Part print with two shaded views. Sizes in mm from the minimum x, y, z corner. Coordinates: 2 decimals unless noted, no trailing zeros. Order: outer loops, then holes, each group sorted by start corner. A loop starts at its lowest first (then second) coordinate and runs counter-clockwise, first axis right, second up.
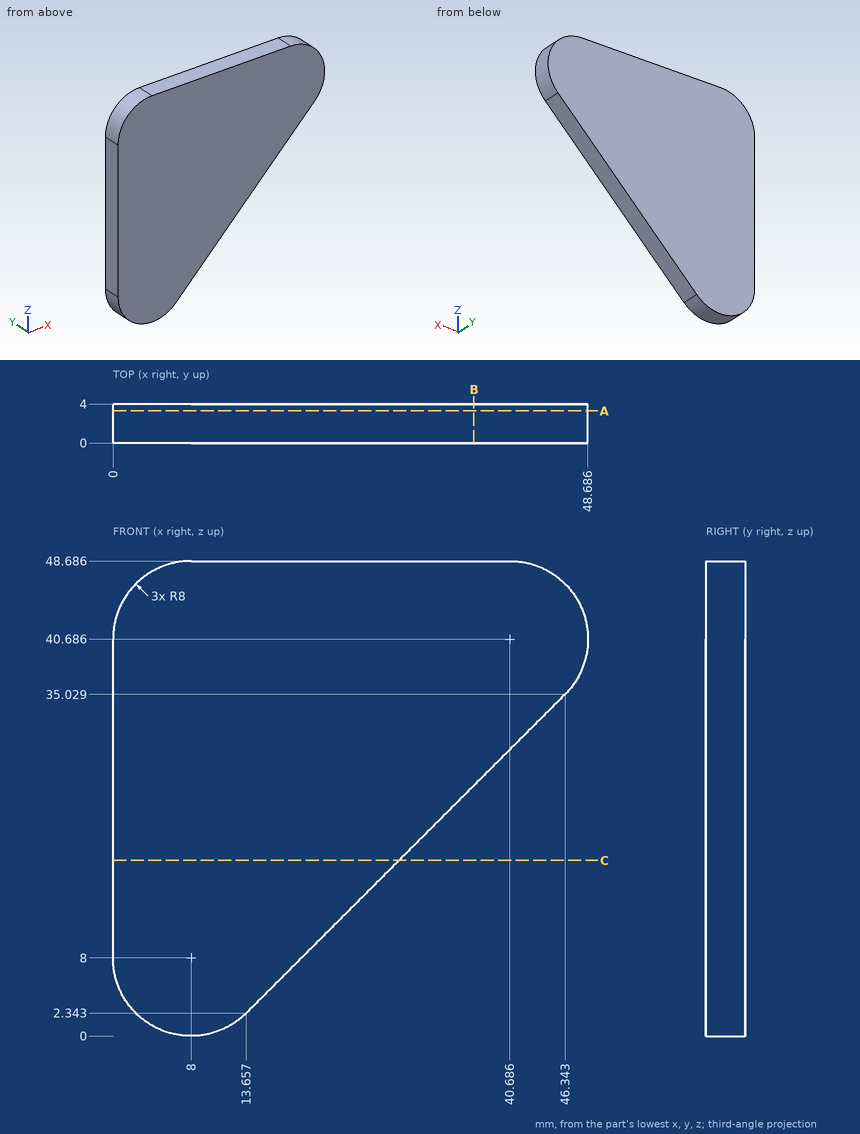
Q1. Wall check: line 1 along X through (y, z) = (3.2, 41); line 2 along Z through (x, y) = (19, 1.35) (1 decimal); line 3 along X through (y, z) = (1.65, 18) (1 decimal). Give the ranges that are in metal, low to high.
Results list:
line 1: x = 0.01 to 48.68
line 2: z = 7.7 to 48.7
line 3: x = 0 to 29.3
Q2. Cut at C-C on z = 18. Write the cut outline in (x, y).
Results list:
outline: (0, 0) - (29.31, 0) - (29.31, 4) - (0, 4) - close
Q3. Cut at B-B on x = 37. Write the cut outline in (y, z), and give its area (3 significant figures).
Results list:
outline: (0, 25.69) - (4, 25.69) - (4, 48.69) - (0, 48.69) - close
area: 92.0 mm2
Q4. Cut at A-A on y = 3.3. Write the cut outline in (x, z).
Results list:
outline: (0, 8) arc R8 ccw to (13.66, 2.34) - (46.34, 35.03) arc R8 ccw to (40.69, 48.69) - (8, 48.69) arc R8 ccw to (0, 40.69) - close
Q5. Pin check, flat tips, straight feed: pin 1 Ø1 at (y, z) = (1, 43.5) entering from -X; pin 2 Ø2 at (x, y) = (17.5, 1) entering from -Z (1 decimal). Stop position of each tip, or through.
Results list:
pin 1: stops at x = 0.34
pin 2: stops at z = 5.2
